from build123d import *

# Parameters (mm, degrees)
ESBO_O1_R                = 4.25
RESSALTO_EXTRUS_O1_DEPTH = 6
ESBO_O2_W                = 1.5
ESBO_O2_H                = 20
CORTE_EXTRUS_O1_DEPTH    = 25.5


with BuildPart() as part:
    # Esboço1 → Ressalto-extrusão1 (new body)
    with BuildSketch(Plane.XY):
        with BuildLine():
            ThreePointArc((-78.750627195, 41.976919217), (-92.874182887, 42.196130929), (-100, 30))
            Line((-100, 30), (-100, -4.2))
            Line((-100, -4.2), (-78, -4.2))
            Line((-78, -4.2), (-78, -10))
            Line((-78, -10), (-48, -10))
            Line((-48, -10), (-48, -4.2))
            Line((-48, -4.2), (48, -4.2))
            Line((48, -4.2), (48, -10))
            Line((48, -10), (78, -10))
            Line((78, -10), (78, -4.2))
            Line((78, -4.2), (100, -4.2))
            Line((100, -4.2), (100, 30))
            ThreePointArc((100, 30), (92.874182887, 42.196130929), (78.750627195, 41.976919217))
            ThreePointArc((78.750627195, 41.976919217), (0, 20), (-78.750627195, 41.976919217))
        make_face()
        with Locations((-86, 30)):
            Circle(ESBO_O1_R, mode=Mode.SUBTRACT)
        with Locations((86, 30)):
            Circle(ESBO_O1_R, mode=Mode.SUBTRACT)
    extrude(amount=RESSALTO_EXTRUS_O1_DEPTH)

    # Esboço2 → Corte-extrusão1 (cut)
    with BuildSketch(Plane.XY.offset(6)):
        with Locations((-39.8, 2.8)):
            Rectangle(ESBO_O2_W, ESBO_O2_H)
        with Locations((39.8, 2.8)):
            Rectangle(ESBO_O2_W, ESBO_O2_H)
    extrude(amount=-CORTE_EXTRUS_O1_DEPTH, mode=Mode.SUBTRACT)


solid = part.part
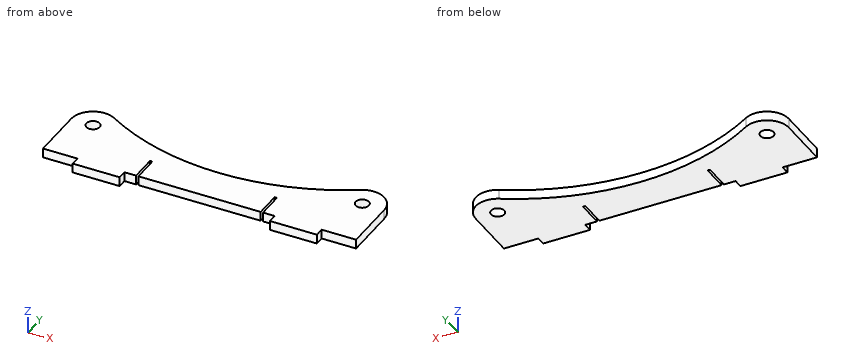
Check sheet for the modelled part. Datum: model origin and axes. Units: mm. Round coordinates to 2 decimals unless told otherwise and drop trailing zeros. Loops run counter-clockwise (first coordinate to the right, second up) from the corner with the lowest first, then second, coordinate; pieces in that order, holes last. Notation, with made-up numbers: M 9,76 L 24,76 A29 ccw 24,107 Z; hole C -40,74 d4. An arc over 180 degrees is marked long. One line per item, written item: value.
(1) Sectioned sample at B-B, the plane y = -1.5. Record the cut outline in (x, z), then the cut area to 3 significant figures.
Computed values:
outline: M -100,0 L -40.55,0 L -40.55,6 L -100,6 Z; M -39.05,0 L 39.05,0 L 39.05,6 L -39.05,6 Z; M 40.55,0 L 100,0 L 100,6 L 40.55,6 Z
area: 1,180 mm^2
(2) Depth check by flat-ended pin: pin 1 Ø1.6 at (x, z) = (40, 2) entering from -Y; pin 2 Ø1.7 at (y, z) = (-6.5, 3.5) entering from +X; pin 3 Ø0.8 at (x, z) = (-40, 4.5) entering from -Y. Enter the tip coordinate at first touch or a pass-through.
Computed values:
pin 1: stops at y = -4.2
pin 2: stops at x = 78
pin 3: stops at y = 12.8
(3) Thickness scan on line 1 (X direction, y = 8, z = 2.8); line 2 (X direction, y = 31.5, z = 0.8); line 3 (Y direction, x = -86, z = 1.3). Record the ranges inside material, lowest first.
Computed values:
line 1: x = -100 to -40.55, -39.05 to 39.05, 40.55 to 100
line 2: x = -99.92 to -89.98, -82.02 to -58.01, 58.01 to 82.02, 89.98 to 99.92
line 3: y = -4.2 to 25.75, 34.25 to 44
(4) Sectioned sample at D-D, the plane y = 38.5. Record the cut outline in (x, z).
Computed values:
outline: M -97.12,0 L -72.7,0 L -72.7,6 L -97.12,6 Z; M 72.7,0 L 97.12,0 L 97.12,6 L 72.7,6 Z
(5) Sectioned sample at C-C, the plane x = -86. Record the cut outline in (y, z), then the cut area to 3 significant figures.
Computed values:
outline: M -4.2,0 L 25.75,0 L 25.75,6 L -4.2,6 Z; M 34.25,0 L 44,0 L 44,6 L 34.25,6 Z
area: 238 mm^2
(6) Sectioned sample at A-A, the plane z = 3.4. Record the cut outline in (x, y).
Computed values:
outline: M -100,-4.2 L -78,-4.2 L -78,-10 L -48,-10 L -48,-4.2 L -40.55,-4.2 L -40.55,12.8 L -39.05,12.8 L -39.05,-4.2 L 39.05,-4.2 L 39.05,12.8 L 40.55,12.8 L 40.55,-4.2 L 48,-4.2 L 48,-10 L 78,-10 L 78,-4.2 L 100,-4.2 L 100,30 A14 ccw 78.75,41.98 A152.08 cw -78.75,41.98 A14 ccw -100,30 Z; hole C -86,30 d8.5; hole C 86,30 d8.5
